Model file for the job. Use its own axes, mm. Coordinates: 2 decimals unless noted, no trailing zeros. Loops run counter-clockwise (first coordinate to the right, second up) from the corner with the lowest first, then second, coordinate; pieces in that order, holes last.
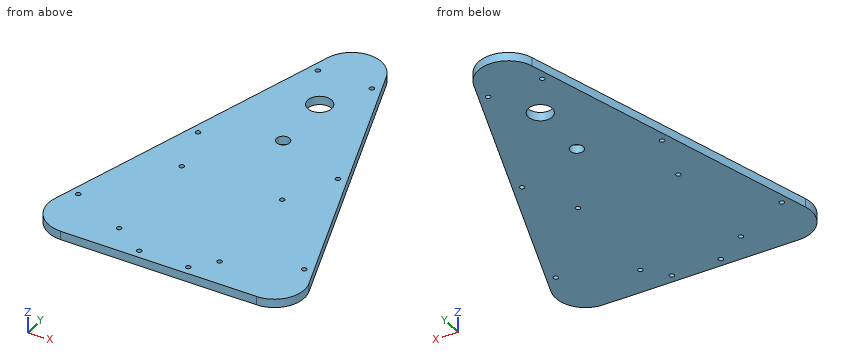
Autodesk Inventor part; units mm, degrees
ref_plane "Work Plane1" through (0, 0, 4.572) normal (0, 0, 1) x (1, 0, 0)
ref_plane "YZ Plane" through (0, 0, 0) normal (1, 0, 0) x (0, 1, 0)
ref_plane "XZ Plane" through (0, 0, 0) normal (0, 1, 0) x (-1, 0, 0)
sketch "Sketch1" plane through (0, 0, 0) normal (0, 0, 1) x (1, 0, 0)
  arc A0 (-2.400661, 17.597517) -> (12.7, -3.175) centre (12.7, 12.7) ccw
  arc A1 (114.3, -3.175) -> (129.400661, 17.597517) centre (114.3, 12.7) ccw
  line L0 (114.3, -3.175) -> (12.7, -3.175)
  line L1 (48.399339, 174.230681) -> (-2.400661, 17.597517)
  line L2 (129.400661, 17.597517) -> (78.600661, 174.230681)
  arc A2 (78.600661, 174.230681) -> (48.399339, 174.230681) centre (63.5, 169.333164) ccw
  arc A3 (75.580529, 173.251177) -> (51.419471, 173.251177) centre (63.5, 169.333164) ccw
  arc A4 (0.619471, 16.618013) -> (12.7, 0) centre (12.7, 12.7) ccw
  arc A5 (114.3, 0) -> (126.380529, 16.618013) centre (114.3, 12.7) ccw
  line L3 (12.7, 0) -> (114.3, 0)
  line L4 (0.619471, 16.618013) -> (51.419471, 173.251177)
  line L5 (75.580529, 173.251177) -> (126.380529, 16.618013)
  line L6 (0.619471, 16.618013) -> (3.753882, 26.282436)
  line L7 (3.753882, 26.282436) -> (4.961935, 25.890635)
  circle A6 centre (4.961935, 25.890635) radius 1.27
  line L8 (51.419471, 173.251177) -> (48.285061, 163.586755)
  line L9 (48.285061, 163.586755) -> (49.493113, 163.194953)
  circle A7 centre (49.493113, 163.194953) radius 1.27
  circle A8 centre (27.227524, 94.542794) radius 1.27
  line L10 (75.580529, 173.251177) -> (78.714939, 163.586755)
  line L11 (78.714939, 163.586755) -> (77.506886, 163.194953)
  circle A9 centre (77.506886, 163.194953) radius 1.27
  line L12 (126.380529, 16.618013) -> (123.246118, 26.282436)
  line L13 (123.246118, 26.282436) -> (122.038065, 25.890635)
  circle A10 centre (122.038065, 25.890635) radius 1.27
  circle A11 centre (99.772476, 94.542794) radius 1.27
  line L14 (63.5, 0) -> (63.5, 1.27) construction
  line L15 (63.5, 1.27) -> (76.2, 1.27) construction
  line L16 (63.5, 1.27) -> (50.8, 1.27) construction
  circle A12 centre (50.8, 1.27) radius 1.27
  circle A13 centre (76.2, 1.27) radius 1.27
  point P0 (0, 0)
  point P1 (0, 0)
  dimension "d50" = 2.54
  dimension "d53" = 2.54
  dimension "d39" = 31.75
  dimension "d40" = 31.75
  dimension "d41" = 25.4
  dimension "d42" = 25.4
  dimension "d43" = 25.4
  dimension "d44" = 10.16
  dimension "d45" = 10.16
  dimension "d46" = 1.27
  dimension "d47" = 1.27
  dimension "d48" = 10.16
  dimension "d49" = 10.16
  dimension "d51" = 2.54
  dimension "d52" = 2.54
  dimension "d91" = 12.7
  dimension "d92" = 12.7
ref_plane "Work Plane1" through (0, 0, 4.572) normal (0, 0, 1) x (1, 0, 0)
sketch "Sketch2" plane through (0, 0, 4.572) normal (0, 0, 1) x (1, 0, 0)
  line L0 (12.7, -3.175) -> (114.3, -3.175)
  line L1 (34.171935, 12.065) -> (34.171935, 67.945) construction
  line L2 (34.171935, 67.945) -> (86.241935, 67.945) construction
  line L3 (86.241935, 67.945) -> (86.241935, 12.065) construction
  line L4 (86.241935, 12.065) -> (34.171935, 12.065) construction
  line L5 (34.171935, 12.065) -> (86.241935, 67.945) construction
  line L6 (34.171935, 67.945) -> (86.241935, 12.065) construction
  circle A0 centre (34.171935, 67.945) radius 1.27
  circle A1 centre (34.171935, 12.065) radius 1.27
  circle A2 centre (86.241935, 12.065) radius 1.27
  circle A3 centre (86.241935, 67.945) radius 1.27
  circle A4 centre (4.961935, 25.890635) radius 1.27
  circle A5 centre (63.5, 140.758164) radius 6.35
  arc A6 (78.600661, 174.230681) -> (48.399339, 174.230681) centre (63.5, 169.333164) ccw
  circle A7 centre (63.5, 108.090258) radius 3.429
  point P0 (0, 0)
  point P1 (60.206935, 40.005)
  dimension "d71" = 55.88
  dimension "d73" = 52.07
  dimension "d74" = 2.54
  dimension "d75" = 2.54
  dimension "d76" = 2.54
  dimension "d77" = 2.54
  dimension "d80" = 52.07
  dimension "d81" = 15.24
  dimension "d82" = 29.21
  dimension "d84" = 12.7
  dimension "d87" = 38.1
  dimension "d88" = 6.858
sketch "Sketch1 outline for Extrusion8" plane through (0, 0, 0) normal (0, 0, 1) x (1, 0, 0)
  arc A0 (78.600661, 174.230681) -> (48.399339, 174.230681) centre (63.5, 169.333164) ccw
  line L0 (129.400661, 17.597517) -> (78.600661, 174.230681)
  line L1 (48.399339, 174.230681) -> (-2.400661, 17.597517)
  arc A1 (114.3, -3.175) -> (129.400661, 17.597517) centre (114.3, 12.7) ccw
  arc A2 (-2.400661, 17.597517) -> (12.7, -3.175) centre (12.7, 12.7) ccw
  line L2 (12.7, -3.175) -> (114.3, -3.175)
  circle A3 centre (4.961935, 25.890635) radius 1.27
  circle A4 centre (50.8, 1.27) radius 1.27
  circle A5 centre (76.2, 1.27) radius 1.27
  circle A6 centre (122.038065, 25.890635) radius 1.27
  circle A7 centre (27.227524, 94.542794) radius 1.27
  circle A8 centre (49.493113, 163.194953) radius 1.27
  circle A9 centre (99.772476, 94.542794) radius 1.27
  circle A10 centre (77.506886, 163.194953) radius 1.27
extrude "Extrusion8" add sketch "Sketch1 outline for Extrusion8" along normal blind 4.572
extrude "Extrusion9" cut sketch "Sketch2" against normal blind 4.572 contours A0 | A1 | A2 | A3 | A5 | A7
properties part number "Nathan_LED_Speaker_Back"
Q1. Slice it at D-D (x = 42). List the corners of the cut face in (y, z) (3 decimals).
Answers:
outline: (-3.175, 0) - (154.499, 0) - (154.499, 4.572) - (-3.175, 4.572) - close
Q2. Drill centre lines: line 1 (Y direction, x = 63.5, z = 1.65) (3 decimals); line 2 (X direction, y = 13, z = 4.3); line 3 (X direction, y = 25, z = 2.05). Where is each one in solid material? Low to high.
Answers:
line 1: y = -3.175 to 104.661, 111.519 to 134.408, 147.108 to 185.208
line 2: x = -3.17 to 33.31, 35.03 to 85.38, 87.1 to 130.17
line 3: x = 0 to 4.06, 5.87 to 121.13, 122.94 to 127
Q3. Slice it at C-C (z = 2.7). Count the separate pieces of the cut face and the enclosed holes in it, and give its area (3 significant figures).
Answers:
separate pieces: 1
enclosed holes: 14
area: 15,400 mm2
Q4. Slice it at B-B (x = 63.5). List the corners of the cut face in (y, z) (3 decimals), and give its area (3 significant figures).
Answers:
outline: (-3.175, 0) - (104.661, 0) - (104.661, 4.572) - (-3.175, 4.572) - close; (111.519, 0) - (134.408, 0) - (134.408, 4.572) - (111.519, 4.572) - close; (147.108, 0) - (185.208, 0) - (185.208, 4.572) - (147.108, 4.572) - close
area: 772 mm2
Q5. Flat gauge pins, fed straight in: P1, Ø1.5, axis at y = 81.5, z = 1, coming from the -X side; P2, Ø1.5, axis at x = 53.5, z = 3, coming from the +Y side; P3, Ø2, axis at x = 78.5, z = 4, coming from the +Y side. Where does each tip first touch, or does it go through?
Answers:
P1: stops at x = 18.08
P2: stops at y = 182.23
P3: stops at y = 176.82
Q6. Slice it at A-A (y = 137). List the corners of the cut face in (x, z), and give its area (3 significant figures).
Answers:
outline: (36.32, 0) - (58.38, 0) - (58.38, 4.57) - (36.32, 4.57) - close; (68.62, 0) - (90.68, 0) - (90.68, 4.57) - (68.62, 4.57) - close
area: 202 mm2
